Geometry: final body of the model. Coordinates: model frame, mm. A direction names the side the tool comes from. Round coordinates to 2 decimals unless told otherwise and drop trailing zeros. Write each loop counter-clockwise with the first axis right and the second up, starting at its lowest first coordinate (ties: lowest second). Pieces come first, ordered by that corner, then holes. Notation, with made-up numbers: M 79.5,80 L 103.5,80 A26 cw 103.5,95 Z; hole C -0.5,65.25 d7. An arc over 180 degrees is marked long. Answer as CSV lines item,"result". Start each with the question number.
Q1. Ray query, probe 1 along Z at (x, y) = (1, -13.5); probe 2 along X at (y, z) = (0, -7); probe 3 along Y at (x, z) = (0, 13). Return the intervals inside material, ascending.
Q2. Section query C-C on z = 52. Output: boundary loops of the cut face in (x, y), and give its area (3 significant figures).
Q3. Section query A-A on x = 0. Output: boundary loops of the cut face in (y, z), and give its area (3 significant figures).
Q4. Reachability of faces 1 (the flat face through (0, 2, -7)), 2 (the cylindrical face through (-0.1, -2.5, -6.9)), 3 (the flat face through (0, 0, 70)) from +Z, -Z, +X, -X, +Y, -Y: full face, straight path, thin tool, end or side. Return the list, or none.
Q5. First-contact query: pin 1 (1 mm diameter, centred on y = 7.5, z = 38, fed in from -X); pin 2 (10 mm diameter, centred on y = 12.5, z = 18.5, fed in from -X); pin 3 (12 mm diameter, centred on y = 10.5, z = 21.5, fed in from +X). Flat tips, straight axial feed; report the tip coordinate or a pass-through.
Q6. Section query D-D on z = -4.5. Output: boundary loops of the cut face in (x, y).
Q7. Section query B-B on y = 0. Output: boundary loops of the cut face in (x, z).
```python
from build123d import *

# Parameters (mm, degrees)
SKETCH1_R           = 18
BOSS_EXTRUDE1_DEPTH = 70
BOSS_EXTRUDE2_DEPTH = 14
FILLET1_R           = 2


with BuildPart() as part:
    # Sketch1 → Boss-Extrude1 (new body)
    with BuildSketch(Plane.XY):
        Circle(SKETCH1_R)
    extrude(amount=BOSS_EXTRUDE1_DEPTH)

    # Sketch2 → Boss-Extrude2 (add)
    with BuildSketch(Plane(origin=(0, 0, 0), x_dir=(-1, 0, 0), z_dir=(0, 0, -1))):
        with BuildLine():
            Line((-1.5, 2), (1.5, 2))
            ThreePointArc((1.5, 2), (0, -2.5), (-1.5, 2))
        make_face()
    extrude(amount=BOSS_EXTRUDE2_DEPTH)

    # Fillet1
    fillet1_edges = [part.edges().sort_by_distance(p)[0] for p in [
        (-18, 0, 0),
        (-18, 0, 70),
    ]]
    fillet(fillet1_edges, radius=FILLET1_R)


solid = part.part
```
Entries:
1,probe 1,"z = 0 to 70"
1,probe 2,"x = -2.5 to 2.5"
1,probe 3,"y = -18 to 18"
2,outline,"C 0,0 d36"
2,area,"1,020 mm^2"
3,outline,"M -18,2 A2 ccw -16,0 L -2.5,0 L -2.5,-14 L 2,-14 L 2,0 L 16,0 A2 ccw 18,2 L 18,68 A2 ccw 16,70 L -16,70 A2 ccw -18,68 Z"
3,area,"2,580 mm^2"
4,face 1,"-Z, +X, -X, +Y"
4,face 2,"-Z"
4,face 3,"+Z, +X, -X, +Y, -Y"
5,pin 1,"stops at x = -16.58"
5,pin 2,"stops at x = -16.36"
5,pin 3,"stops at x = 17.43"
6,outline,"M -1.5,2 A2.5 ccw long 1.5,2 Z"
7,outline,"M -18,2 A2 ccw -16,0 L -2.5,0 L -2.5,-14 L 2.5,-14 L 2.5,0 L 16,0 A2 ccw 18,2 L 18,68 A2 ccw 16,70 L -16,70 A2 ccw -18,68 Z"
